Build history of the part. All positions in model axes, mm. A direction names the side the tool comes from. Give positions to 0.01 mm unless a question says otherwise; leave off trailing zeros. Order: outer loops, then holes, each group sorted by start corner. A loop starts at its lowest first (then second) coordinate and runs counter-clockwise, first axis right, second up. Notation, with made-up numbers: (23, -3) -> (37, -3) arc R22 cw to (37, 6) -> close; hole circle Ø4 at (2.5, -28.5). An arc over 180 degrees is marked (long way). One line per question, with ' | ' between items. Start each with the question number.
(1) Cut at A-A (x = -17.5). Give the cut face in (y, z).
(2) Pin check, flat tips, straight feed: pin 1 Ø1.8 at (x, y) = (25.5, 13) entering from +Z; pin 2 Ø3 at (x, y) = (26, -11.5) entering from +Z; pin 3 Ø6 at (x, y) = (22.5, -2) entering from +Z. Stop position of each tip, or through.
(3) Drill centre lines: L1, parallel to X at y = -5, z = 3.6; L2, parallel to Y at x = 14.5, z = 3.95; L3, parallel to Y at x = -24.75, z = 0.95. Where is each one in solid material? Low to high. Write a range as from..to.
(4) Pull direction X, two halves, no side cores. Call faces 4 (the face through (15.467, 14, 2)), 5 (the face through (0, -17.5, 2)), 6 (the face through (-29.75, 0, 2)): +X half, -X half, draft (parallel to the pull), parting line (faces both ways), or undercut.
(5) Which spindle directions (+Z, -Z, +X, -X, +Y, -Y) get a long thin tool onto all of the face, cutting with end or side? Do faces 1 (the face through (0, 17.5, 2)), 2 (the face through (8, 8.9, 3)), 3 (the face through (-3.467, -14, 2)). Say none if no direction does.
(6) Cut at B-B (z = 3.4). Give the number of separate pieces and of enclosed holes in the cut face, then the cut area to 3 significant figures.
Autodesk Inventor part; units mm, degrees
ref_plane "YZ Plane" through (0, 0, 0) normal (1, 0, 0) x (0, 1, 0)
ref_plane "XZ Plane" through (0, 0, 0) normal (0, 1, 0) x (-1, 0, 0)
ref_plane "XY Plane" through (0, 0, 0) normal (0, 0, 1) x (1, 0, 0)
sketch "スケッチ1" plane through (0, 0, 0) normal (0, 0, 1) x (1, 0, 0)
  line L0 (29.75, 17.5) -> (29.75, -17.5)
  line L1 (29.75, -17.5) -> (-29.75, -17.5)
  line L2 (-29.75, -17.5) -> (-29.75, 17.5)
  line L3 (-29.75, 17.5) -> (29.75, -17.5) construction
  line L4 (29.75, 17.5) -> (-29.75, -17.5) construction
  line L5 (-3.4667, -15.05) -> (-1.3667, -15.05) construction
  line L6 (15.4667, -15.05) -> (15.4667, -12.45)
  line L7 (15.4667, -12.45) -> (13.3667, -12.45) construction
  line L8 (-3.4667, -12.45) -> (-3.4667, -15.05)
  line L9 (-3.4667, -15.05) -> (15.4667, -12.45) construction
  line L10 (15.4667, -15.05) -> (-3.4667, -12.45) construction
  line L11 (-3.4167, -12.5) -> (15.4167, -12.5) construction
  line L12 (15.4167, -12.5) -> (15.4167, -15) construction
  line L13 (15.4167, -15) -> (-3.4167, -15) construction
  line L14 (-3.4167, -15) -> (-3.4167, -12.5) construction
  line L15 (-3.4167, -12.5) -> (15.4167, -15) construction
  line L16 (15.4167, -12.5) -> (-3.4167, -15) construction
  arc A0 (-1.3667, -12.45) -> (-3.4667, -12.45) centre (-2.4167, -12.45) ccw
  line L17 (-3.4667, -13.75) -> (15.4667, -13.75) construction
  arc A1 (-3.4667, -15.05) -> (-1.3667, -15.05) centre (-2.4167, -15.05) ccw
  line L18 (-1.3667, -12.45) -> (-3.4667, -12.45) construction
  line L19 (-1.3667, -15.05) -> (13.3667, -15.05)
  line L20 (13.3667, -12.45) -> (-1.3667, -12.45)
  line L21 (13.3667, -15.05) -> (15.4667, -15.05) construction
  line L22 (-29.75, 17.5) -> (29.75, 17.5)
  line L23 (6, 17.5) -> (6, -17.5) construction
  line L24 (-29.75, 0) -> (29.75, 0) construction
  arc A2 (15.4667, -12.45) -> (13.3667, -12.45) centre (14.4167, -12.45) ccw
  arc A3 (13.3667, -15.05) -> (15.4667, -15.05) centre (14.4167, -15.05) ccw
  line L25 (-3.4667, 15.05) -> (-1.3667, 15.05) construction
  line L26 (15.4667, 15.05) -> (15.4667, 12.45)
  line L27 (15.4667, 12.45) -> (13.3667, 12.45) construction
  line L28 (-3.4667, 12.45) -> (-3.4667, 15.05)
  line L29 (-3.4667, 15.05) -> (15.4667, 12.45) construction
  line L30 (15.4667, 15.05) -> (-3.4667, 12.45) construction
  line L31 (-3.4167, 12.5) -> (15.4167, 12.5) construction
  line L32 (15.4167, 12.5) -> (15.4167, 15) construction
  line L33 (15.4167, 15) -> (-3.4167, 15) construction
  line L34 (-3.4167, 15) -> (-3.4167, 12.5) construction
  line L35 (-3.4167, 12.5) -> (15.4167, 15) construction
  line L36 (15.4167, 12.5) -> (-3.4167, 15) construction
  arc A4 (-3.4667, 12.45) -> (-1.3667, 12.45) centre (-2.4167, 12.45) ccw
  line L37 (-3.4667, 13.75) -> (15.4667, 13.75) construction
  arc A5 (-1.3667, 15.05) -> (-3.4667, 15.05) centre (-2.4167, 15.05) ccw
  line L38 (-1.3667, 12.45) -> (-3.4667, 12.45) construction
  line L39 (-1.3667, 15.05) -> (13.3667, 15.05)
  line L40 (13.3667, 12.45) -> (-1.3667, 12.45)
  line L41 (13.3667, 15.05) -> (15.4667, 15.05) construction
  arc A6 (15.4667, 15.05) -> (13.3667, 15.05) centre (14.4167, 15.05) ccw
  arc A7 (13.3667, 12.45) -> (15.4667, 12.45) centre (14.4167, 12.45) ccw
  circle A8 centre (25.4167, -12.5) radius 1.6
  circle A9 centre (25.4167, -12.5) radius 3
  circle A10 centre (25.4167, 12.5) radius 1.6
  circle A11 centre (25.4167, 12.5) radius 3
  circle A12 centre (-24.75, 12.5) radius 1.6
  circle A13 centre (-24.75, 12.5) radius 3
  line L42 (-5.9667, -15) -> (-5.9667, -8.9)
  line L43 (-5.9667, -8.9) -> (21.2585, -8.9)
  line L44 (27.25, -7.3146) -> (27.25, 7.3146)
  line L45 (-19.851, 15) -> (-5.9167, 15)
  arc A14 (-21.15, 8.3419) -> (-19.851, 15) centre (-24.75, 12.5) ccw
  line L46 (-27.25, 2.5) -> (-24.75, 2.5) construction
  line L47 (-24.75, 2.5) -> (-24.75, -7.5) construction
  line L48 (-24.75, -7.5) -> (-27.25, -7.5) construction
  line L49 (-27.25, -7.5) -> (-27.25, 2.5) construction
  line L50 (-27.25, 2.5) -> (-24.75, -7.5) construction
  line L51 (-24.75, 2.5) -> (-27.25, -7.5) construction
  line L52 (-27.3, 2.55) -> (-24.7, 2.55)
  line L53 (-24.7, 2.55) -> (-24.7, -7.55)
  line L54 (-24.7, -7.55) -> (-27.3, -7.55)
  line L55 (-27.3, -7.55) -> (-27.3, 2.55)
  line L56 (-27.3, 2.55) -> (-24.7, -7.55) construction
  line L57 (-24.7, 2.55) -> (-27.3, -7.55) construction
  arc A15 (-27.3, 2.55) -> (-27.3, 0.45) centre (-27.3, 1.5) ccw
  line L58 (-26, 2.55) -> (-26, -7.55) construction
  line L59 (-27.3, -2.5) -> (-24.7, -2.5) construction
  arc A16 (-24.7, 0.45) -> (-24.7, 2.55) centre (-24.7, 1.5) ccw
  arc A17 (-27.3, -5.45) -> (-27.3, -7.55) centre (-27.3, -6.5) ccw
  arc A18 (-24.7, -7.55) -> (-24.7, -5.45) centre (-24.7, -6.5) ccw
  line L60 (-21.15, 8.3419) -> (-21.15, -15)
  line L61 (-5.9667, 15) -> (-5.9667, 8.9)
  line L62 (-21.15, -15) -> (-5.9667, -15)
  arc A19 (27.25, -7.3146) -> (21.2585, -8.9) centre (25.4167, -12.5) ccw
  line L63 (-5.9667, 8.9) -> (21.2585, 8.9)
  arc A20 (21.2585, 8.9) -> (27.25, 7.3146) centre (25.4167, 12.5) ccw
  point P0 (0, 0)
  point P1 (6, -13.75)
  point P2 (6, -13.75)
  point P3 (6, -13.75)
  point P4 (6, 13.75)
  point P5 (6, 13.75)
  point P6 (6, 13.75)
  point P7 (-26, -2.5)
  point P8 (-27.3, -5.45)
  point P9 (-24.7, 0.45)
  point P10 (-24.7, -5.45)
  point P11 (-5.9667, 15)
  point P12 (27.25, 7.3146)
  dimension "d0" = 59.5
  dimension "d1" = 35
  dimension "d6" = 18.8333
  dimension "d7" = 0.05
  dimension "d8" = 0.05
  dimension "d9" = 1.05
  dimension "d26" = 35.75
  dimension "d27" = 5
  dimension "d31" = 3.2
  dimension "d32" = 6
  dimension "d33" = 5
  dimension "d34" = 10
  dimension "d39" = 5
  dimension "d40" = 5
  dimension "d41" = 3.2
  dimension "d42" = 6
  dimension "d43" = 2.5
  dimension "d50" = 2.5
  dimension "d51" = 2.5
  dimension "d54" = 2.5
  dimension "d56" = 2.5
  dimension "d60" = 1.05
  dimension "d61" = 0.05
  dimension "d62" = 0.05
  dimension "d63" = 2.5
  dimension "d64" = 2.5
  dimension "d65" = 10
  dimension "d68" = 2.5
  dimension "d71" = 2.5
  dimension "d75" = 10
  dimension "d76" = 2.5
  dimension "d77" = 2.5
extrude "押し出し1" add sketch "スケッチ1" along normal blind 5 contours L0 L1 L2 L22
extrude "押し出し2" add sketch "スケッチ1" along normal blind 2 contours A9 | A11 | A13
chamfer "面取り1" distance 2.5 angle 45 4 edges at (-29.75, 17.5, 2.5) (-29.75, -17.5, 2.5) (29.75, 17.5, 2.5) (29.75, -17.5, 2.5)
extrude "押し出し3" add sketch "スケッチ1" along normal blind 1 contours L62 L60 A14 L45 L61 L63 A20 L44 A19 L43 L42
fillet "フィレット1" radius 1 11 edges at (-19.851, 15, 3) (-21.15, 8.3419, 3) (-5.9667, -8.9, 3) (-5.9667, 15, 3) (-5.9667, -15, 3) (-21.15, -15, 3) (21.2585, 8.9, 3) (27.25, 7.3146, 3) (27.25, -7.3146, 3) (21.2585, -8.9, 3) (-5.9667, 8.9, 3)
equation "\"d6\" = d4"
equation "\"d8\" = d7"
equation "\"d41\" = d31"
equation "\"d42\" = d32"
equation "\"d50\" = d49"
equation "\"d60\" = d9"
equation "\"d61\" = d7"
equation "\"d62\" = d61"
properties part number "Cockpit_vertical_frame_05" material "アセタール樹脂、黒"
Result set:
1) outline: (-17.5, 0) -> (17.5, 0) -> (17.5, 5) -> (15, 5) -> (15, 1) -> (-15, 1) -> (-15, 5) -> (-17.5, 5) -> close
2) pin 1: passes through | pin 2: stops at z = 2 | pin 3: stops at z = 1
3) L1: x = -29.75..-27.3, -24.7..-21.15, 27.25..29.75 | L2: y = -17.5..-16.1, -11.4..-8.9, 8.9..11.4, 16.1..17.5 | L3: y = -17.5..-7.55, 2.55..10.9, 14.1..17.5
4) face 4: undercut | face 5: draft | face 6: -X half
5) face 1: +Z, -Z, +X, -X, +Y | face 2: +Z | face 3: +Z, -Z
6) separate pieces: 1 | enclosed holes: 7 | area: 822 mm2
